```python
from build123d import *

# Parameters (mm, degrees)
BOSS_EXTRUDE1_DEPTH      = 150
BOSS_EXTRUDE1_DEPTH_BACK = 150
CHAMFER1_SIZE            = 0.225


with BuildPart() as part:
    # Sketch3 → Boss-Extrude1 (new body, two sides)
    with BuildSketch(Plane.XY) as boss_extrude1_sk:
        with BuildLine():
            Line((-2.5, 4.071067812), (-2.5, 7.071067812))
            ThreePointArc((-2.5, 7.071067812), (0, -7.5), (2.5, 7.071067812))
            Line((2.5, 7.071067812), (2.5, 4.071067812))
            Line((2.5, 4.071067812), (-2.5, 4.071067812))
        make_face()
    extrude(amount=BOSS_EXTRUDE1_DEPTH)
    extrude(boss_extrude1_sk.sketch, amount=-BOSS_EXTRUDE1_DEPTH_BACK)

    # Chamfer1
    chamfer1_edges = [part.edges().sort_by_distance(p)[0] for p in [
        (0, -7.5, -150),
        (0, -7.5, 150),
    ]]
    chamfer(chamfer1_edges, length=CHAMFER1_SIZE)


solid = part.part
```
The listing builds one solid part. Answer for the finished solid, in the listing's coordinates (mm). Give positions to 0.01 mm unless a question says otherwise; leave off trailing zeros. Order: outer loops, then holes, each group sorted by start corner. A loop starts at its lowest first (then second) coordinate and runs counter-clockwise, first axis right, second up. Notation, with made-up numbers: (64, 22.5) - (112, 22.5) arc R14 ccw to (112, 34.5) - close; hole circle Ø8 at (57, 64). An arc over 180 degrees is marked (long way). Answer in a Markdown table with one row per item. Add a question column.
Q1. The part is cut by section A-A (x = 0). Determine the outline of the cut face in (y, z) (3 decimals).
Q2. Find the intervals of material crossed by line 1 along Y through (x, z) = (-0.5, 101.5); line 2 along Y through (x, z) = (-2, -0.5); line 3 along X through (y, z) = (0.75, -95), in increasing order. Write a range as [from, to].
Q3. The part is cut by section B-B (z = 30.5). Determine the outline of the cut face in (x, y).
Q4. For a pull along X with two mould halves and no side action, classify faces 1 (the flat face through (0, 0, -150)), 2 (the flat face through (0, 4.071, 2)), 3 (the conical face through (-0.29, -7.38, -149.89)) as released by +X, released by -X, zero draft, split by the parting line, or undercut.
Q5. Given P1, Ø3.5, axis at y = 6.5, z = -11.5, coming from the -X side; P2, Ø1, axis at y = -2, z = -63, coming from the -X side; P3, Ø1, axis at x = -4, z = 38.5, coming from the -Y side, each flat-ended and moving along its own axis, determine where each tip first touches the part or whether it passes through.
Determined:
| question | item | result |
|---|---|---|
| 1 | outline | (-7.5, -149.775) - (-7.275, -150) - (4.071, -150) - (4.071, 150) - (-7.275, 150) - (-7.5, 149.775) - close |
| 2 | line 1 | y = [-7.48, 4.07] |
| 2 | line 2 | y = [-7.23, 4.07] |
| 2 | line 3 | x = [-7.46, 7.46] |
| 3 | outline | (-2.5, 4.07) - (-2.5, 7.07) arc R7.5 ccw (long way) to (2.5, 7.07) - (2.5, 4.07) - close |
| 4 | face 1 | zero draft |
| 4 | face 2 | undercut |
| 4 | face 3 | split by the parting line |
| 5 | P1 | stops at x = -5.8 |
| 5 | P2 | stops at x = -7.35 |
| 5 | P3 | stops at y = -6.63 |
